Autodesk Inventor part; units mm, degrees
ref_plane "Arbeitsebene1" through (0, 0, -3) normal (0, 0, 1) x (1, 0, 0)
ref_plane "YZ Plane" through (0, 0, 0) normal (1, 0, 0) x (0, 1, 0)
ref_plane "XZ Plane" through (0, 0, 0) normal (0, 1, 0) x (-1, 0, 0)
sketch "Skizze1" plane through (0, 0, 0) normal (0, 0, 1) x (1, 0, 0)
  circle A0 centre (0, 0) radius 7.5
  circle A1 centre (0, 0) radius 4
  dimension "d0" = 15
  dimension "d3" = 8
extrude "Extrusion1" add sketch "Skizze1" against normal blind 14
ref_plane "Arbeitsebene1" through (0, 0, -3) normal (0, 0, 1) x (1, 0, 0)
sketch "Skizze2" plane through (0, 0, -3) normal (0, 0, 1) x (1, 0, 0)
  circle A0 centre (-15, 0) radius 5
  circle A1 centre (15, 0) radius 5
  circle A2 centre (-15, 0) radius 2.8
  circle A3 centre (15, 0) radius 2.8
  point P0 (0, 0)
  dimension "d5" = 10
  dimension "d6" = 10
  dimension "d7" = 15
  dimension "d8" = 15
  dimension "d9" = 5.6
  dimension "d10" = 5.6
extrude "Extrusion2" add sketch "Skizze2" against normal blind 14
sketch "Skizze3" plane through (-15, 0, -3) normal (0, 0, 1) x (1, 0, 0)
  circle A0 centre (0, 0) radius 5
  circle A1 centre (0, 0) radius 2.8
  circle A2 centre (15, 0) radius 7.5
  circle A3 centre (15, 0) radius 4
  circle A4 centre (30, 0) radius 5
  circle A5 centre (30, 0) radius 2.8
  circle A6 centre (15, 0) radius 7.5
  line L0 (-5.1094, 4.2073) -> (15, 7.6064)
  line L1 (15, 7.6064) -> (38.7432, 3.5931)
  circle A7 centre (30, 0) radius 5
  line L2 (-7.8587, -3.7426) -> (15, -7.6064)
  line L3 (15, -7.6064) -> (39.1845, -3.5185)
  point P0 (16.25, -7.3951)
  point P1 (30.8333, -4.9301)
  point P2 (30.8333, 4.9301)
  point P3 (16.25, 7.3951)
  point P4 (-0.8333, -4.9301)
  point P5 (13.75, -7.3951)
  point P6 (13.75, 7.3951)
  point P7 (-0.8333, 4.9301)
extrude "Extrusion3" add sketch "Skizze3" against normal blind 11 contours A0 L0 A2 L2 | L1 A4 L3 A2
properties part number "250_CameraMount"
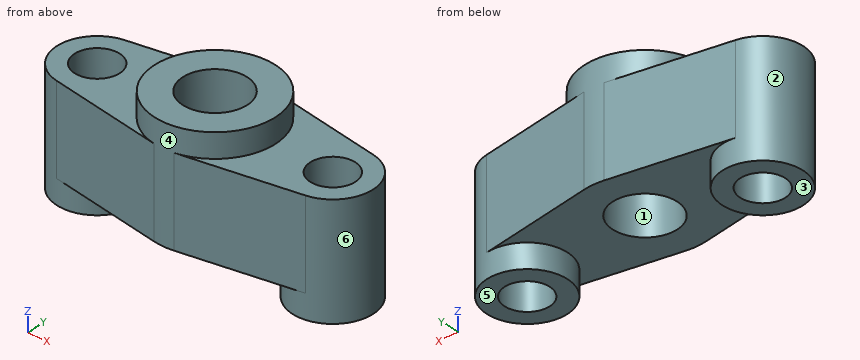
Input: part model. Units: mm. Frame: model coordinates. Face numbers are marked on the shaded views. A direction names the side the tool comes from. Give positions to 0.01 mm unless a question says otherwise; leave off trailing zeros. Loops run counter-clockwise (first coordinate to the right, second up) from the corner with the lowest first, then second, coordinate; pieces in that order, holes last. Notation, with made-up numbers: (56.25, -39.5) - (72.25, -39.5) arc R27 cw to (72.25, -22.5) - close; hole circle Ø11 at (17, 22). An arc over 180 degrees is marked (long way). Use CSV: the item, a comma, the result in double quotes. Start each with the question number.
Item 1: Section C-C on z = -2.25. Return loops of the section in (x, y).
Item 2: Contact query for flat-ended pins moving along their axis: P1, Ø3, axis at y = 3, z = -3.5, coming from the -X side; P2, Ø1, axis at y = -3, z = -4, coming from the -X side. Output: stop coordinate, or through.
Item 3: Reachability of the marked faces 4, 5 and 6 from +Z, -Z, +X, -X, +Y, -Y: full face, straight path, thin tool, end or side. Return the list, or none.
Item 4: Section B-B on y = -3.5. Return loops of the section in (x, z).
Item 5: Mould query, pull axis Y, two halves, no side actions, for the marked faces 1, 2 and 3. Classes: pulls with the +Y half, pulls with the -Y half, needs draft (parallel to the pull), parting line crosses it, or undercut.
Item 6: Section A-A on x = 0. Return loops of the section in (y, z).
Item 7: Line query: line 1 (X direction, y = 0.75, z = -5.25); line 2 (Y direction, x = 0, z = -8); line 3 (Z direction, x = 18, y = -3). Output: solid intervals per line, ascending.
Item 8: Section D-D on z = -8.25. Return loops of the section in (x, y).
Ans:
1,outline,"circle Ø15 at (0, 0); hole circle Ø8 at (0, 0)"
2,P1,"stops at x = -19.77"
2,P2,"stops at x = -19.33"
3,face 4,"+Z"
3,face 5,"-Z, +X, -X, +Y, -Y"
3,face 6,"-Z"
4,outline,"(-18.57, -17) - (-11.43, -17) - (-11.43, -14) - (-1.94, -14) - (-1.94, 0) - (-6.63, 0) - (-6.63, -3) - (-18.57, -3) - close; (1.94, -14) - (11.43, -14) - (11.43, -17) - (18.57, -17) - (18.57, -3) - (6.63, -3) - (6.63, 0) - (1.94, 0) - close"
5,face 1,"undercut"
5,face 2,"parting line crosses it"
5,face 3,"needs draft"
6,outline,"(-7.5, -14) - (-4, -14) - (-4, 0) - (-7.5, 0) - close; (4, -14) - (7.5, -14) - (7.5, 0) - (4, 0) - close"
7,line 1,"x = -19.94 to -17.7, -12.3 to -3.93, 3.93 to 12.3, 17.7 to 19.94"
7,line 2,"y = -7.5 to -4, 4 to 7.5"
7,line 3,"z = -17 to -3"
8,outline,"(-15.83, -4.93) - (-1.25, -7.4) arc R7.5 ccw to (1.25, -7.4) - (15.83, -4.93) arc R5 ccw to (15.83, 4.93) - (1.25, 7.4) arc R7.5 ccw to (-1.25, 7.4) - (-15.83, 4.93) arc R5 ccw to start; hole circle Ø5.6 at (-15, 0); hole circle Ø8 at (0, 0); hole circle Ø5.6 at (15, 0)"
